Build history of the part. All positions in model axes, mm. A direction names the side the tool comes from. Give positions to 0.01 mm unless a question says otherwise; leave off trailing zeros. Loops run counter-clockwise (first coordinate to the right, second up) from the corner with the lowest first, then second, coordinate; pieces in that order, holes last. Notation, with made-up numbers: M 64.25,37 L 91.25,37 A33 ccw 91.25,69 Z; hole C 22.5,81 d11. An arc over 180 degrees is marked long. Put each result on its own line as item: value.
```python
from build123d import *

# Parameters (mm, degrees)
SKETCH1_R           = 8.5
BOSS_EXTRUDE1_DEPTH = 2
SKETCH2_R           = 4.3
BOSS_EXTRUDE2_DEPTH = 6
SKETCH3_R           = 8.5
BOSS_EXTRUDE3_DEPTH = 2
SKETCH4_R           = 4
CUT_EXTRUDE1_DEPTH  = 2
SKETCH5_R           = 2
CUT_EXTRUDE2_DEPTH  = 11
FILLET1_R           = 1


with BuildPart() as part:
    # Sketch1 → Boss-Extrude1 (new body)
    with BuildSketch(Plane(origin=(0, 0, 0), x_dir=(1, 0, 0), z_dir=(0, 1, 0))):
        Circle(SKETCH1_R)
    extrude(amount=BOSS_EXTRUDE1_DEPTH)

    # Sketch2 → Boss-Extrude2 (add)
    with BuildSketch(Plane(origin=(0, 2, 0), x_dir=(1, 0, 0), z_dir=(0, 1, 0))):
        Circle(SKETCH2_R)
    extrude(amount=BOSS_EXTRUDE2_DEPTH)

    # Sketch3 → Boss-Extrude3 (add)
    with BuildSketch(Plane(origin=(0, 8, 0), x_dir=(1, 0, 0), z_dir=(0, 1, 0))):
        Circle(SKETCH3_R)
    extrude(amount=BOSS_EXTRUDE3_DEPTH)

    # Sketch4 → Cut-Extrude1 (cut)
    with BuildSketch(Plane(origin=(0, 10, 0), x_dir=(1, 0, 0), z_dir=(0, 1, 0))):
        Circle(SKETCH4_R)
    extrude(amount=-CUT_EXTRUDE1_DEPTH, mode=Mode.SUBTRACT)

    # Sketch5 → Cut-Extrude2 (cut)
    with BuildSketch(Plane(origin=(0, 8, 0), x_dir=(1, 0, 0), z_dir=(0, 1, 0))):
        Circle(SKETCH5_R)
    extrude(amount=-CUT_EXTRUDE2_DEPTH, mode=Mode.SUBTRACT)

    # Fillet1
    fillet1_edges = [part.edges().sort_by_distance(p)[0] for p in [
        (-4.3, 2, 0),
        (-4.3, 8, 0),
    ]]
    fillet(fillet1_edges, radius=FILLET1_R)


solid = part.part
```
Q1. Slice it at D-D (x = -6.75). List the corners of the cut face in (y, z), and give its area (3 significant figures).
Here are the results:
outline: M 0,-5.17 L 2,-5.17 L 2,5.17 L 0,5.17 Z; M 8,-5.17 L 10,-5.17 L 10,5.17 L 8,5.17 Z
area: 41.3 mm²
Q2. Probe line 1 (Y direction, x = 2.5, z = 4.75); line 2 (X direction, y = 3.75, z = 0); line 3 (X direction, y = 9.3, z = 0). List the from-to ranges inside material, lowest first. Write a range as from..to.
Here are the results:
line 1: 0..2, 8..10
line 2: -4.3..-2, 2..4.3
line 3: -8.5..-4, 4..8.5
Q3. Tool access for faces 5 (the cylindrical face through (-0.867, 9.014, 3.905)), 6 (the flat face through (4, 2, -4)), 7 (the cylindrical face through (4.57, 0.986, -7.167)): list every direction of +Z, -Z, +X, -X, +Y, -Y with a clear straight run to the whole face (end or side of a thin tool).
Here are the results:
face 5: +Y
face 6: none
face 7: +Y, -Y
Q4. Slice it at A-A (x = 0). List the corners of the cut face in (y, z), and give its area (3 significant figures).
Here are the results:
outline: M 0,-8.5 L 2,-8.5 L 2,-5.3 A1 cw 3,-4.3 L 7,-4.3 A1 cw 8,-5.3 L 8,-8.5 L 10,-8.5 L 10,-4 L 8,-4 L 8,-2 L 0,-2 Z; M 0,2 L 8,2 L 8,4 L 10,4 L 10,8.5 L 8,8.5 L 8,5.3 A1 cw 7,4.3 L 3,4.3 A1 cw 2,5.3 L 2,8.5 L 0,8.5 Z
area: 72.5 mm²
Q5. Slice it at B-B (z = 0). List the corners of the cut face in (x, y), and give its area (3 significant figures).
Here are the results:
outline: M -8.5,0 L -2,0 L -2,8 L -4,8 L -4,10 L -8.5,10 L -8.5,8 L -5.3,8 A1 cw -4.3,7 L -4.3,3 A1 cw -5.3,2 L -8.5,2 Z; M 2,0 L 8.5,0 L 8.5,2 L 5.3,2 A1 cw 4.3,3 L 4.3,7 A1 cw 5.3,8 L 8.5,8 L 8.5,10 L 4,10 L 4,8 L 2,8 Z
area: 72.5 mm²
Q6. Drop flat-ended pins along their axis: pin 1 Ø1 at (x, y) = (2.5, 3) entering from +Z; pin 2 Ø3 at (x, y) = (-3, 8.5) entering from +Z; pin 3 Ø4 at (x, z) = (-1.5, 0) entering from +Y. Give the stop position or say it passes through.
Here are the results:
pin 1: z = 3.81
pin 2: z = 8.37
pin 3: y = 8
Q7. Mould opens along Y. For faces 1 (the flat face through (-2, 8, 1)), 2 (the flat face through (2, 0, 2)), 3 (the cylindrical face through (0, 4, 2)), 4 (the flat face through (4, 8, -4)) say: pulls with the +Y half, pulls with the -Y half, needs draft (parallel to the pull), parting line crosses it, or undercut.
Here are the results:
face 1: pulls with the +Y half
face 2: pulls with the -Y half
face 3: needs draft
face 4: undercut
Q8. Slice it at C-C (z = -6.5). List the corners of the cut face in (x, y), and give its area (3 significant figures).
Here are the results:
outline: M -5.48,0 L 5.48,0 L 5.48,2 L -5.48,2 Z; M -5.48,8 L 5.48,8 L 5.48,10 L -5.48,10 Z
area: 43.8 mm²
